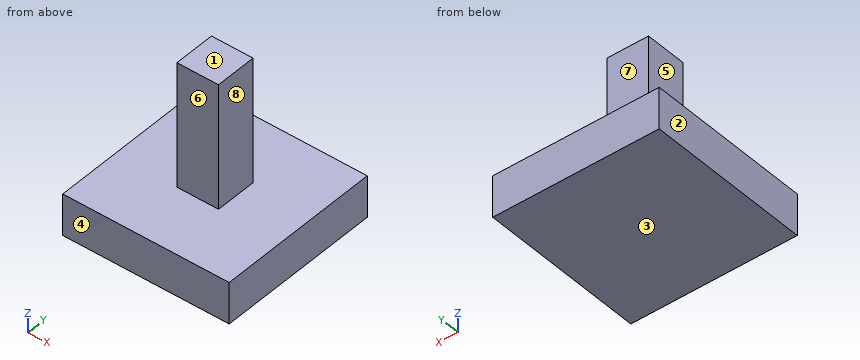
```python
from build123d import *

# Parameters (mm, degrees)
F0_W     = 50.8
F0_H     = 50.8
F1_DEPTH = 12.7
F2_W     = 12.7
F2_H     = 12.7
F3_DEPTH = 50.8


with BuildPart() as f1:
    # F0 (on Top) → F1 (new body)
    with BuildSketch(Plane.XY):
        Rectangle(F0_W, F0_H)
    extrude(amount=F1_DEPTH)

    # F2 (on Top) → F3 (join)
    with BuildSketch(Plane.XY):
        Rectangle(F2_W, F2_H)
    extrude(amount=F3_DEPTH)


solid = f1.part
```
Geometry: final body of the model. Coordinates: model frame, mm. Face numbers are marked on the shaded views. A direction names the side the tool comes from. Round coordinates to 2 decimals unless told otherwise and drop trailing zeros. Write each loop counter-clockwise with the first axis right and the second up, starting at its lowest first coordinate (ties: lowest second). Pieces come first, ordered by that corner, then holes.
Item 1: Section query C-C (z = 34). Return loops of the section in (x, y).
Item 2: Section query A-A (x = 1). Return loops of the section in (y, z), plus the area to 3 significant figures.
Item 3: Set-up query: the marked faces 4, 5, 6, 7 and 8. Return all of +Z, -Z, +X, -X, +Y, -Y with unobstructed straight access to the full face (end or side cutting, diameter ignored); none if empty.
Item 4: Pin query (flat end, axial travel): P1, Ø3, axis at x = -14.5, z = 13.5, coming from the -Y side; P2, Ø10, axis at y = 0, z = 30, coming from the -X side; P3, Ø14, axis at x = -1, z = 23, coming from the +Y side; P4, Ø14, axis at y = 2.5, z = 25.5, coming from the +X side. Return the tip coordinate at first contact, or that it passes through.
Item 5: Section query D-D (x = -18.5). Return loops of the section in (y, z), plus the area to 3 significant figures.
Item 6: Material intervals for L1, parallel to Z at x = -21, y = -12; L2, parallel to Y at x = 3, z = 25.5, sorted ascending.
Item 7: Mould query, pull axis Z, two halves, no side actions, for the marked faces 1, 2 and 3. Classes: +Z half, -Z half, draft (parallel to the pull), parting line (faces both ways), or undercut.
Completed:
1. outline: (-6.35, -6.35) - (6.35, -6.35) - (6.35, 6.35) - (-6.35, 6.35) - close
2. outline: (-25.4, 0) - (25.4, 0) - (25.4, 12.7) - (6.35, 12.7) - (6.35, 50.8) - (-6.35, 50.8) - (-6.35, 12.7) - (-25.4, 12.7) - close
2. area: 1,130 mm2
3. face 4: +Z, -Z, +X, -X, -Y
3. face 5: +Z, -X, +Y, -Y
3. face 6: +Z, +X, -X, -Y
3. face 7: +Z, +X, -X, +Y
3. face 8: +Z, +X, +Y, -Y
4. P1: stops at y = -25.4
4. P2: stops at x = -6.35
4. P3: stops at y = 6.35
4. P4: stops at x = 6.35
5. outline: (-25.4, 0) - (25.4, 0) - (25.4, 12.7) - (-25.4, 12.7) - close
5. area: 645 mm2
6. L1: z = 0 to 12.7
6. L2: y = -6.35 to 6.35
7. face 1: +Z half
7. face 2: draft
7. face 3: -Z half
